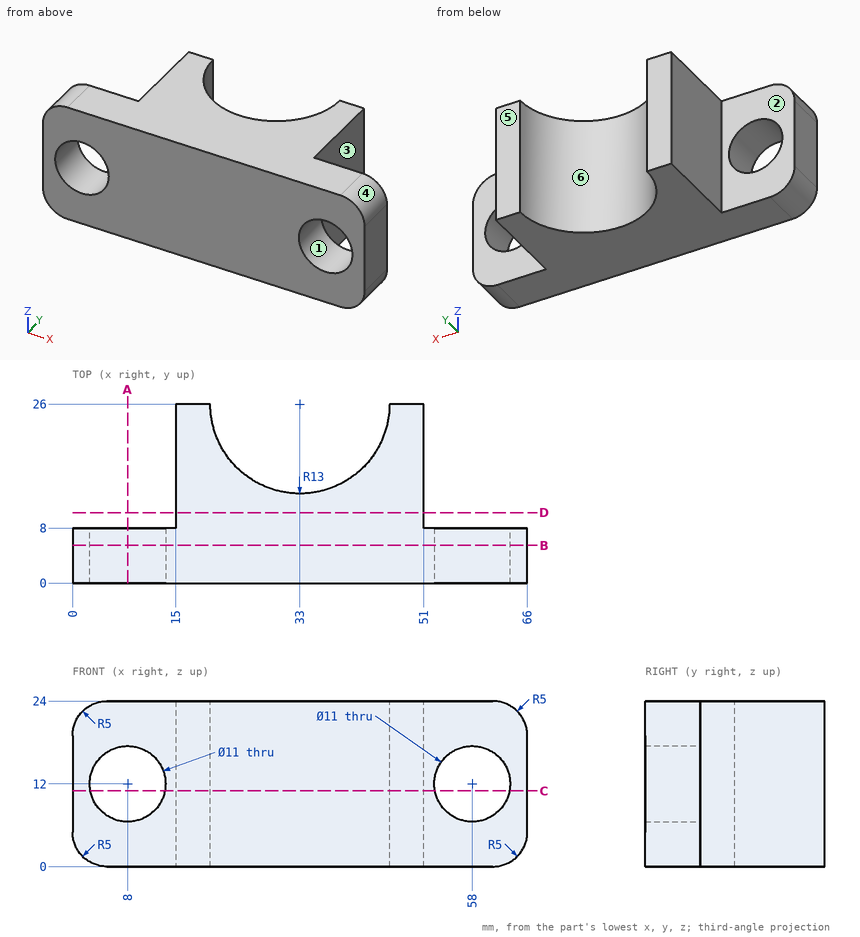
Drawing for the job (mm, zero at the part's lowest x, y, z). A direction names the side the tool comes from. Give positions to 0.01 mm unless a question says otherwise; leave off trailing zeros. Write each loop counter-clockwise with the first axis right and the second up, starting at its lowest first coordinate (ties: lowest second). Pieces come first, ordered by that corner, then holes. Notation, with made-up numbers: M -6,54 L 9,54 A20 ccw 9,76 Z; hole C 1,71 d5. An arc over 180 degrees is marked long. Return JSON: item names as keys, results as strings. Group by question number.
(1) 3-axis set-ups, long thin cutter, end or side, ignore diameter. For the marked faces 1, 2 and 3: which of +Z, -Z, +X, -X, +Y, -Y reach the whole face in a straight line?
(2) Band-saw the part on C-C (z = 11). Give the cut face in (x, y), and give its area (3 significant figures).
(3) Mould opens along X. For the marked faces 4, 5 and 6 say: pulls with the +X half, pulls with the -X half, needs draft (parallel to the pull), parting line crosses it, or undercut.
(4) Band-saw the part on D-D (y = 10.25). Give the cut face in (x, z).
(5) Flat gauge pins, fed straight in: pin 1 Ø1.5 at (y, z) = (12, 17) entering from -X; pin 2 Ø1 at (x, z) = (17, 4.5) entering from -Y; pin 3 Ø4.5 at (x, z) = (6, 16.5) entering from +Y; pin 4 Ø10 at (y, z) = (20.5, 10) entering from +X. Where does each tip first touch, or does it go through?
(6) Band-saw the part on A-A (x = 8). Give the cut face in (y, z), and give its area (3 significant figures).
(7) Band-saw the part on B-B (y = 5.5). Give the cut face in (x, z), and give its area (3 significant figures).
(8) Drill centre lines: L1, parallel to Z at x = 58, y = 4.25; L2, parallel to X at y = 9.5, z = 11.25; L3, parallel to Y at x = 10, z = 22.25. Where is each one in solid material? Low to high. Write a range as [from, to].
Entries:
{
 "1": {"face 1": "+Y, -Y", "face 2": "+Z, -Z, -X, +Y", "face 3": "+Z, -Z, +X, +Y"},
 "2": {"outline": "M 0,0 L 2.59,0 L 2.59,8 L 0,8 Z; M 13.41,0 L 52.59,0 L 52.59,8 L 51,8 L 51,26 L 46,26 A13 cw 20,26 L 15,26 L 15,8 L 13.41,8 Z; M 63.41,0 L 66,0 L 66,8 L 63.41,8 Z", "area": "737 mm^2"},
 "3": {"face 4": "pulls with the +X half", "face 5": "needs draft", "face 6": "undercut"},
 "4": {"outline": "M 15,0 L 51,0 L 51,24 L 15,24 Z"},
 "5": {"pin 1": "stops at x = 15", "pin 2": "stops at y = 0", "pin 3": "stops at y = 8", "pin 4": "stops at x = 51"},
 "6": {"outline": "M 0,0 L 8,0 L 8,6.5 L 0,6.5 Z; M 0,17.5 L 8,17.5 L 8,24 L 0,24 Z", "area": "104 mm^2"},
 "7": {"outline": "M 0,5 A5 ccw 5,0 L 61,0 A5 ccw 66,5 L 66,19 A5 ccw 61,24 L 5,24 A5 ccw 0,19 Z; hole C 8,12 d11; hole C 58,12 d11", "area": "1,370 mm^2"},
 "8": {"L1": "z = [0, 6.5], [17.5, 24]", "L2": "x = [15, 51]", "L3": "y = [0, 8]"}
}
